Input: part model. Units: mm. Frame: model coordinates. A direction names the side the tool comes from. Give positions to 0.01 mm unless a question says otherwise; leave off trailing zeros. Order: outer loops, then holes, each group sorted by start corner. A loop starts at its lowest first (then second) coordinate and runs counter-clockwise, first axis right, second up. Notation, with made-up numbers: (-16, -27) - (28, -27) arc R26 ccw to (28, 6) - close; hole circle Ø11 at (29, 86). An arc over 180 degrees is marked (long way). Use a Markdown table: item, result.
from build123d import *


with BuildPart() as f1:
    # F0 (on Top) → F1 (revolve)
    with BuildSketch(Plane.XY):
        with BuildLine():
            ThreePointArc((0, -65.188989), (18.207665, -66.653242), (34.861051, -74.15843))
            ThreePointArc((34.861051, -74.15843), (42.039067, -73.239244), (42.199682, -66.004395))
            Line((42.199682, -66.004395), (42.199682, 61.1986))
            Line((42.199682, 61.1986), (31.599436, 61.1986))
            Line((31.599436, 61.1986), (31.599436, 66.091023))
            Line((31.599436, 66.091023), (25.076205, 66.091023))
            Line((25.076205, 66.091023), (25.076205, 61.1986))
            Line((25.076205, 61.1986), (0, 61.1986))
            Line((0, 61.1986), (0, -65.188989))
        make_face()
    revolve(axis=Axis((0, -3.626004, 0), (0, -1, 0)))


solid = f1.part
1. Material intervals for line 1 along Z through (x, y) = (0, 64); line 2 along Z through (x, y) = (1.5, 7.5); line 3 along Y through (x, z) = (-24.5, 28.5), sorted ascending.
Response:
| item | result |
|---|---|
| line 1 | z = -31.6 to -25.08, 25.08 to 31.6 |
| line 2 | z = -42.17 to 42.17 |
| line 3 | y = -75.07 to 61.2 |
2. Pin query (flat end, axial travel): pin 1 (12 mm diameter, centred on x = 33.5, y = 51, fed in from -Z); pin 2 (5 mm diameter, centred on y = 50.5, z = 33, fed in from +X); pin 3 (6 mm diameter, centred on y = -2.5, z = 26, fed in from +X). Return the tip coordinate at first contact, or that it passes through.
Response:
| item | result |
|---|---|
| pin 1 | stops at z = -32.01 |
| pin 2 | stops at x = 29.16 |
| pin 3 | stops at x = 35.38 |
3. Set-up query: faces 1 (the face through (0, 61.199, 0)), 2 (the face through (-19, 66.091, 17)). Return all of +Z, -Z, +X, -X, +Y, -Y with unobstructed straight access to the full face (end or side cutting, diameter ignored); none if empty.
Response:
| item | result |
|---|---|
| face 1 | +Y |
| face 2 | +Z, -Z, +X, -X, +Y |
4. Section query A-A (y = -16). Return loops of the section in (x, z).
Response:
| item | result |
|---|---|
| outline | circle Ø84.4 at (0, 0) |
